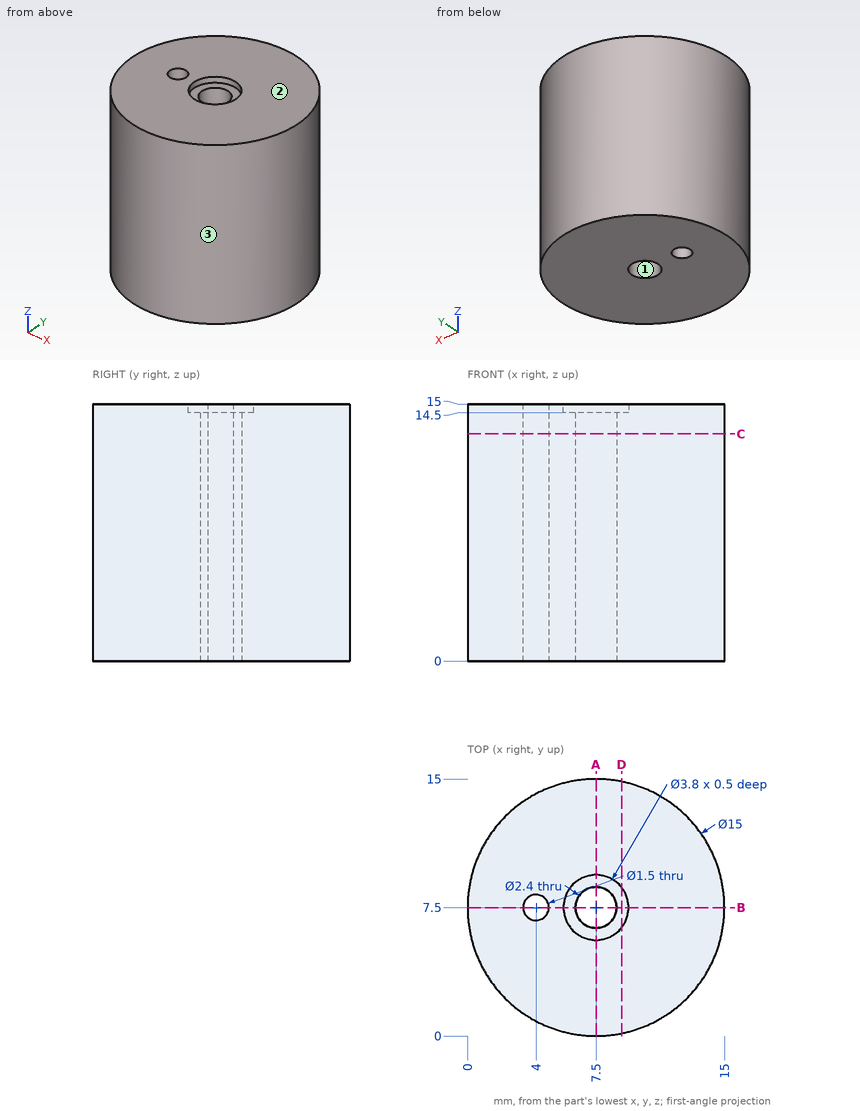
Source: three-view drawing plus pictorial views. Frame: mm from the lowest corner of the part. Give positions to 0.01 mm unless a question says otherwise; leave off trailing zeros. Loops run counter-clockwise (first coordinate to the right, second up) from the corner with the lowest first, then second, coordinate; pieces in that order, holes last.
1) Section query C-C on z = 13.25. Return the cut outline in (x, y), and give its area (3 significant figures).
A:
outline: circle Ø15 at (7.5, 7.5); hole circle Ø1.5 at (4, 7.5); hole circle Ø2.4 at (7.5, 7.5)
area: 170 mm2
2) Section query D-D on x = 9. Return the cut outline in (y, z), and give its area (3 significant figures).
A:
outline: (0.15, 0) - (14.85, 0) - (14.85, 15) - (8.67, 15) - (8.67, 14.5) - (6.33, 14.5) - (6.33, 15) - (0.15, 15) - close
area: 219 mm2
3) Section query B-B on y = 7.5. Return the cut outline in (x, z).
A:
outline: (0, 0) - (3.25, 0) - (3.25, 15) - (0, 15) - close; (4.75, 0) - (6.3, 0) - (6.3, 14.5) - (5.6, 14.5) - (5.6, 15) - (4.75, 15) - close; (8.7, 0) - (15, 0) - (15, 15) - (9.4, 15) - (9.4, 14.5) - (8.7, 14.5) - close
4) Line query: L1, parallel to Y at x = 7.5, z = 14.7; L2, parallel to Y at x = 7.5, z = 10.5; L3, parallel to X at y = 8, z = 2.75. Output: solid intervals per line, ascending.
A:
L1: y = 0 to 5.6, 9.4 to 15
L2: y = 0 to 6.3, 8.7 to 15
L3: x = 0.02 to 3.44, 4.56 to 6.41, 8.59 to 14.98
5) Mould query, pull axis X, two halves, no side actions, for the marked faces 1, 2 and 3. Classes: released by +X, released by -X, zero draft, split by the parting line, or undercut.
A:
face 1: undercut
face 2: zero draft
face 3: split by the parting line
6) Section query A-A on x = 7.5. Return the cut outline in (y, z).
A:
outline: (0, 0) - (6.3, 0) - (6.3, 14.5) - (5.6, 14.5) - (5.6, 15) - (0, 15) - close; (8.7, 0) - (15, 0) - (15, 15) - (9.4, 15) - (9.4, 14.5) - (8.7, 14.5) - close
7) Contact query for flat-ended pins moving along their axis: pin 1 (8 mm diameter, centred on y = 2, z = 7, fed in from -X); pin 2 (2 mm diameter, centred on x = 3.5, z = 2, fed in from +Y); pin 3 (3.5 mm diameter, centred on x = 7.5, y = 7.5, fed in from +Z). Output: stop coordinate, or through.
A:
pin 1: stops at x = 0.15
pin 2: stops at y = 14.37
pin 3: stops at z = 14.5
